Can you work these out from the drawing? Everything is in mm from the part's minimum corner. Round coordinates to 2 decimals unless told otherwise and drop trailing zeros. Write each loop counter-clockwise with the first axis right and the second up, starting at its lowest first coordinate (ties: lowest second). Pieces come first, ordered by that corner, then holes.
Q1. If we section it at B-B (y = 7.25): Please give me the cut outline in (x, z), plus the area to 3 significant figures.
Q2. Please list where these lines run through material, in increasing order: line 1 along X through (y, z) = (7.75, 2.65); line 2 along X through (y, z) = (1.25, 4) (1 decimal); line 3 along X through (y, z) = (5, 35).
Q3. If we section it at D-D (z = 31): Please give me the cut outline in (x, y), plus the area to 3 significant figures.
Q4. If we section it at C-C (x = 82.95): Please give me the cut outline in (y, z), plus the area to 3 significant figures.
Q5. If we section it at A-A (z = 2.65): Please give me the cut outline in (x, y).
Q6. I'm going to push a flat-ended pin straight in: pin 1 Ø2.5 at (x, z) = (82.95, 69.85) entering from +Y. Where does the tip first touch, or does it pass through?
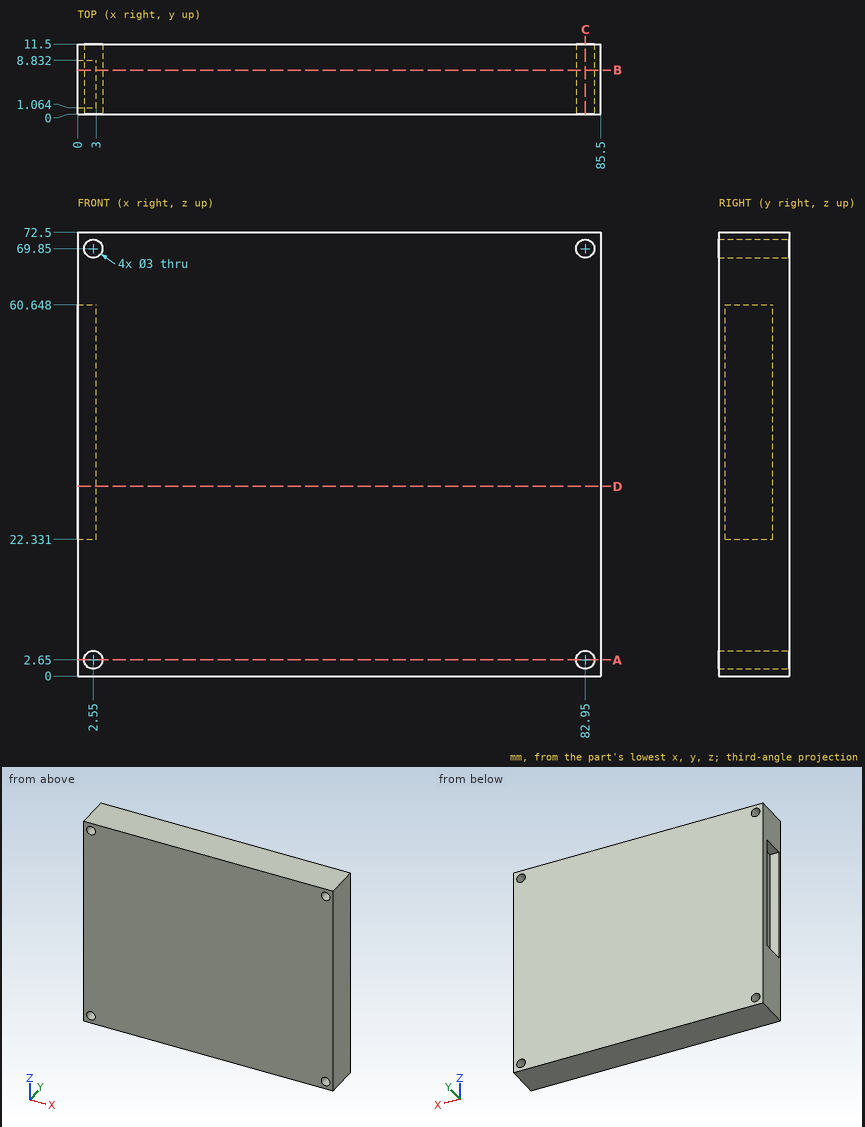
A:
1. outline: (0, 0) - (85.5, 0) - (85.5, 72.5) - (0, 72.5) - (0, 60.65) - (3, 60.65) - (3, 22.33) - (0, 22.33) - close; hole circle Ø3 at (2.55, 2.65); hole circle Ø3 at (2.55, 69.85); hole circle Ø3 at (82.95, 2.65); hole circle Ø3 at (82.95, 69.85)
1. area: 6,060 mm2
2. line 1: x = 0 to 1.05, 4.05 to 81.45, 84.45 to 85.5
2. line 2: x = 0 to 1.9, 3.2 to 82.3, 83.6 to 85.5
2. line 3: x = 3 to 85.5
3. outline: (0, 0) - (85.5, 0) - (85.5, 11.5) - (0, 11.5) - (0, 8.83) - (3, 8.83) - (3, 1.06) - (0, 1.06) - close
3. area: 960 mm2
4. outline: (0, 0) - (11.5, 0) - (11.5, 1.15) - (0, 1.15) - close; (0, 4.15) - (11.5, 4.15) - (11.5, 68.35) - (0, 68.35) - close; (0, 71.35) - (11.5, 71.35) - (11.5, 72.5) - (0, 72.5) - close
4. area: 765 mm2
5. outline: (0, 0) - (1.05, 0) - (1.05, 11.5) - (0, 11.5) - close; (4.05, 0) - (81.45, 0) - (81.45, 11.5) - (4.05, 11.5) - close; (84.45, 0) - (85.5, 0) - (85.5, 11.5) - (84.45, 11.5) - close
6. pin 1: passes through
